Source: CAD feature listing. Evaluate the final solid. Frame: model axes, mm. Face numbers are marked on the shaded views. A direction names the side the tool comes from. Give positions to 0.01 mm unless a question says otherwise; leave off trailing zeros. Loops run counter-clockwise (first coordinate to the right, second up) from the corner with the lowest first, then second, coordinate; pieces in that order, holes last. Notation, with made-up numbers: M 71.25,-18.5 L 129.25,-18.5 A14 cw 129.25,-6.5 Z; hole C 87,28.25 d6. An arc over 180 degrees is marked long. Answer in a Markdown table with one row per item.
```python
from build123d import *

# Parameters (mm, degrees)
SKETCH1_R           = 3.96875
SKETCH1_R_2         = 2
SKETCH1_R_3         = 1.651
SKETCH1_R_4         = 1.559587107
SKETCH1_R_5         = 5.334
BOSS_EXTRUDE1_DEPTH = 8.89


with BuildPart() as part:
    # Sketch1 → Boss-Extrude1 (new body)
    with BuildSketch(Plane(origin=(0, 0, 0), x_dir=(1, 0, 0), z_dir=(0, 1, 0))):
        with BuildLine():
            Line((80.3275, 31.75), (-7.9375, 31.75))
            Line((-7.9375, 31.75), (-7.9375, 13.97))
            Line((-7.9375, 13.97), (-7.9375, 0))
            ThreePointArc((-7.9375, 0), (0, -7.9375), (7.9375, 0))
            Line((7.9375, 0), (15.843955531, 5.536159764))
            Line((15.843955531, 5.536159764), (22.275753266, 5.536159764))
            ThreePointArc((22.275753266, 5.536159764), (36.248751472, 0.907685249), (50.221749679, 5.536159764))
            Line((50.221749679, 5.536159764), (56.546044469, 5.536159764))
            Line((56.546044469, 5.536159764), (64.4525, 0))
            ThreePointArc((64.4525, 0), (72.39, -7.9375), (80.3275, 0))
            Line((80.3275, 0), (80.3275, 13.97))
            Line((80.3275, 13.97), (80.3275, 31.75))
        make_face()
        with Locations(Location((0, 0, 0), (0, 0, 270))):
            Circle(SKETCH1_R, mode=Mode.SUBTRACT)
        with Locations(Location((72.39, 0, 0), (0, 0, 270))):
            Circle(SKETCH1_R, mode=Mode.SUBTRACT)
        with Locations(Location((72.39, 22.86, 0), (0, 0, 270))):
            Circle(SKETCH1_R, mode=Mode.SUBTRACT)
        with Locations(Location((0, 22.86, 0), (0, 0, 270))):
            Circle(SKETCH1_R, mode=Mode.SUBTRACT)
        with Locations(Location((11.43, 8.89, 0), (0, 0, 270))):
            Circle(SKETCH1_R_2, mode=Mode.SUBTRACT)
        with Locations(Location((25.654, 7.822159764, 0), (0, 0, 270))):
            Circle(SKETCH1_R_3, mode=Mode.SUBTRACT)
        with Locations(Location((46.736, 7.822159764, 0), (0, 0, 270))):
            Circle(SKETCH1_R_4, mode=Mode.SUBTRACT)
        with Locations(Location((36.195, 7.822159764, 0), (0, 0, 270))):
            Circle(SKETCH1_R_5, mode=Mode.SUBTRACT)
    extrude(amount=-BOSS_EXTRUDE1_DEPTH)


solid = part.part
```
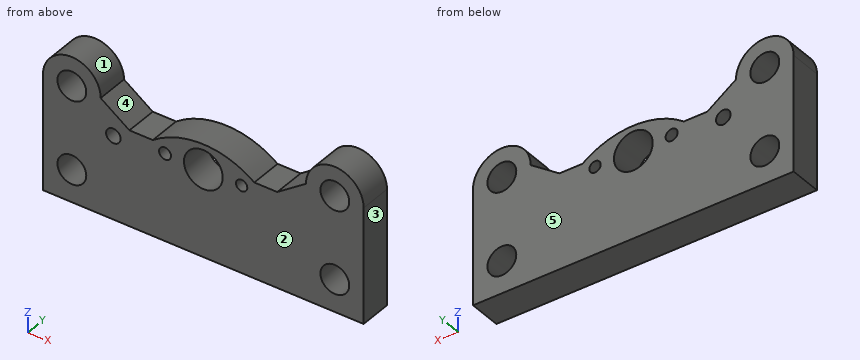
Q1. Section query D-D (x = 11.43). Output: boundary loops of the cut face in (y, z), plus the area to 3 significant figures.
Values follow:
| item | result |
|---|---|
| outline | M -8.89,-31.75 L 0,-31.75 L 0,-10.89 L -8.89,-10.89 Z; M -8.89,-6.89 L 0,-6.89 L 0,-2.45 L -8.89,-2.45 Z |
| area | 225 mm^2 |
Q2. Contact query for flat-ended pins moving along their axis: pin 1 Ø8.5 at (x, z) = (36.2, -7.82) entering from +Y (3 decimals); pin 2 Ø2 at (x, y) = (52.5, -4) entering from +Z. Output: stop coordinate, or through.
Values follow:
| item | result |
|---|---|
| pin 1 | through |
| pin 2 | z = -5.54 |
Q3. Section query B-B (x = 0). Output: boundary loops of the cut face in (y, z), plus the area to 3 significant figures.
Values follow:
| item | result |
|---|---|
| outline | M -8.89,-31.75 L 0,-31.75 L 0,-26.83 L -8.89,-26.83 Z; M -8.89,-18.89 L 0,-18.89 L 0,-3.97 L -8.89,-3.97 Z; M -8.89,3.97 L 0,3.97 L 0,7.94 L -8.89,7.94 Z |
| area | 212 mm^2 |
Q4. Section query A-A (z = -22.86). Output: boundary loops of the cut face in (x, y).
Values follow:
| item | result |
|---|---|
| outline | M -7.94,-8.89 L -3.97,-8.89 L -3.97,0 L -7.94,0 Z; M 3.97,-8.89 L 68.42,-8.89 L 68.42,0 L 3.97,0 Z; M 76.36,-8.89 L 80.33,-8.89 L 80.33,0 L 76.36,0 Z |
Q5. Ray query, probe 1 along X at (y, z) = (-5, -22.5); probe 2 along X at (y, z) = (-2.5, -5); probe 3 along X at (y, z) = (-8, 0.5). Return the intervals inside material, ascending. Write a range as from..to.
Values follow:
| item | result |
|---|---|
| probe 1 | -7.94..-3.95, 3.95..68.44, 76.34..80.33 |
| probe 2 | -7.94..15.08, 23.03..31.67, 40.72..49.47, 57.31..80.33 |
| probe 3 | -7.92..-3.94, 3.94..7.92, 64.47..68.45, 76.33..80.31 |
Q6. Section query C-C (z = -8). Output: boundary loops of the cut face in (x, y), plus the area to 3 significant figures.
Values follow:
| item | result |
|---|---|
| outline | M -7.94,-8.89 L 9.64,-8.89 L 9.64,0 L -7.94,0 Z; M 13.22,-8.89 L 24.01,-8.89 L 24.01,0 L 13.22,0 Z; M 27.3,-8.89 L 30.86,-8.89 L 30.86,0 L 27.3,0 Z; M 41.53,-8.89 L 45.19,-8.89 L 45.19,0 L 41.53,0 Z; M 48.29,-8.89 L 80.33,-8.89 L 80.33,0 L 48.29,0 Z |
| area | 601 mm^2 |
Q7. Mould query, pull axis X, two halves, no side actions, for the marked faces 1, 2 and 3. Classes: +X half, -X half, draft (parallel to the pull), parting line (faces both ways), or undercut.
Values follow:
| item | result |
|---|---|
| face 1 | undercut |
| face 2 | draft |
| face 3 | +X half |
Q8. Reachability of the marked faces 4 and 5 from +Z, -Z, +X, -X, +Y, -Y: full face, straight path, thin tool, end or side. Return the list, or none.
Values follow:
| item | result |
|---|---|
| face 4 | +Z, +Y, -Y |
| face 5 | +Z, -Z, +X, -X, +Y |
